Autodesk Inventor part; units mm, degrees
ref_plane "工作平面2" through (-13.4156, -13.4156, 7) normal (0, 0, 1) x (1, -0.0000484, 0)
ref_plane "工作平面3" through (0, 0, 7) normal (0, 0, 1) x (1, 0, 0)
ref_plane "工作平面4" through (-7.4754, -7.4754, 19) normal (0, 0, 1) x (1, -0.0000484, 0)
sketch "草圖1" plane through (0, 0, 0) normal (0, 0, 1) x (1, 0, 0)
  circle A0 centre (0, 0) radius 19.6
  circle A1 centre (0, 0) radius 41.575
  dimension "d0" = 39.2
  dimension "d1" = 83.15
extrude "擠出1" add sketch "草圖1" along normal blind 5
sketch "草圖2" plane through (0, 0, 0) normal (0, 0, -1) x (-1, 0, 0)
  circle A0 centre (0, 0) radius 41.575
extrude "擠出2" add sketch "草圖2" along normal blind 4
sketch "草圖4" plane through (0, 0, 5) normal (0, 0, 1) x (1, 0, 0)
  circle A0 centre (0, 0) radius 41.575
  circle A1 centre (0, 0) radius 37.575
  dimension "d14" = 4
extrude "擠出4" add sketch "草圖4" along normal blind 47.5
sketch "草圖5" plane through (0, 0, 5) normal (0, 0, 1) x (1, 0, 0)
  circle A0 centre (0, 0) radius 37.575
  circle A1 centre (0, 0) radius 33.075
  dimension "d17" = 4.5
extrude "擠出5" add sketch "草圖5" along normal blind 31.5
sketch "草圖6" plane through (0, 0, -4) normal (0, 0, -1) x (-1, 0, 0)
  line L0 (-66.575, 15.075) -> (-66.575, -15.075)
  line L1 (-66.575, 15.075) -> (-38.7456, 15.075)
  circle A0 centre (0, 0) radius 41.575
  line L2 (-66.575, -15.075) -> (-38.7456, -15.075)
  point P0 (-41.575, 0)
  dimension "d20" = 30.15
  dimension "d22" = 15.075
  dimension "d25" = 25
extrude "擠出6" add sketch "草圖6" against normal up to surface (56.5 mm away) contours L1 A0 L2 L0
sketch "草圖7" plane through (66.575, -15.075, -4) normal (1, 0, 0) x (0, 0, -1)
  line L0 (-56.5, 30.15) -> (-56.5, 0)
  line L1 (0, 0) -> (-56.5, 0)
  line L2 (0, 30.15) -> (0, 0)
  line L3 (0, 30.15) -> (-56.5, 30.15)
  line L4 (-51.5, 5) -> (-31.35, 5)
  line L5 (-31.35, 5) -> (-31.35, 25.15)
  line L6 (-31.35, 25.15) -> (-51.5, 25.15)
  line L7 (-51.5, 25.15) -> (-51.5, 5)
  line L8 (-51.5, 5) -> (-31.35, 25.15) construction
  line L9 (-31.35, 5) -> (-51.5, 25.15) construction
  line L10 (-25.15, 5.0185) -> (-5, 5.0185)
  line L11 (-5, 5.0185) -> (-5, 25.15)
  line L12 (-5, 25.15) -> (-25.15, 25.15)
  line L13 (-25.15, 25.15) -> (-25.15, 5.0185)
  line L14 (-25.15, 5.0185) -> (-5, 25.15) construction
  line L15 (-5, 5.0185) -> (-25.15, 25.15) construction
  point P0 (-4, 15.075)
  point P1 (-41.425, 15.075)
  point P2 (-15.075, 15.0842)
  dimension "d26" = 20.15
  dimension "d27" = 20.15
  dimension "d28" = 20.15
  dimension "d29" = 5
  dimension "d30" = 5
  dimension "d31" = 5
extrude "擠出7" cut sketch "草圖7" against normal blind 20 contours L7 L6 L5 L4 | L13 L12 L11 L10
fillet "圓角1" radius 2 7 edges at (52.6603, 15.075, -4) (-41.575, 0, -4) (52.6603, -15.075, -4) (38.7456, 15.075, 24.25) (52.6603, 15.075, 52.5) (-41.575, 0, 52.5) (52.6603, -15.075, 52.5)
sketch "草圖8" plane through (0, 0, 52.5) normal (0, 0, 1) x (1, 0, 0)
  line L0 (52.9465, -6.0747) -> (44.9865, -6.0635)
  line L1 (52.9465, -6.0747) -> (52.9551, 0.0253)
  line L2 (44.9951, 0.0365) -> (52.9551, 0.0253)
  line L3 (44.9865, -6.0635) -> (44.9951, 0.0365)
  circle A0 centre (48.975, -7.075) radius 2.165
  circle A1 centre (48.975, 7.075) radius 2.165
  line L4 (38.7456, -15.075) -> (66.575, -15.075)
  line L5 (66.575, 15.075) -> (40.0902, 15.075)
  point P0 (0, 0)
  dimension "d36" = 4.33
  dimension "d37" = 4.33
  dimension "d38" = 8
  dimension "d39" = 8
extrude "擠出8" cut sketch "草圖8" against normal up to surface (5 mm away) contours A0 L0 | L0 A0 | A1
sketch "草圖9" plane through (38.7456, -15.075, 50.5) normal (0, -1, 0) x (1, 0, 0)
  line L0 (27.8294, -29.35) -> (27.8294, -49.5)
  line L1 (27.8294, -29.35) -> (7.8294, -29.35)
  line L2 (7.8294, -29.35) -> (7.8294, -49.5)
  line L3 (27.8294, -49.5) -> (7.8294, -49.5)
  line L4 (27.8294, -3) -> (27.8294, -23.15)
  line L5 (27.8294, -3) -> (7.8294, -3)
  line L6 (7.8294, -3) -> (7.8294, -23.15)
  line L7 (27.8294, -23.15) -> (7.8294, -23.15)
  circle A0 centre (17.8294, -39.425) radius 2.1
  circle A1 centre (17.8294, -13.075) radius 2.1
  point P0 (-38.7456, -50.5)
  dimension "d42" = 4.2
  dimension "d43" = 4.2
extrude "擠出9" cut sketch "草圖9" against normal through all contours A0 | A1
sketch "草圖10" plane through (38.7456, -15.075, 50.5) normal (0, -1, 0) x (1, 0, 0)
  circle A0 centre (17.8294, -39.425) radius 2.1
  circle A1 centre (17.8294, -39.425) radius 3.65
  circle A2 centre (17.8294, -13.075) radius 2.1
  circle A3 centre (17.8294, -13.075) radius 3.65
  point P0 (-38.7456, -50.5)
  dimension "d46" = 7.3
  dimension "d47" = 7.3
extrude "擠出10" cut sketch "草圖10" against normal blind 3
mirror "鏡射1" about plane through (0, 0, 0) normal (0, 1, 0) of "擠出10"
sketch "草圖14" plane through (0, 0, 5) normal (0, 0, 1) x (1, 0, 0)
  circle A0 centre (0, 0) radius 19.6
extrude "擠出13" add sketch "草圖14" against normal up to surface (9 mm away)
sketch "草圖15" plane through (0, 0, -4) normal (0, 0, -1) x (-1, 0, 0)
  circle A0 centre (0, 0) radius 13.5
  dimension "d64" = 27
extrude "擠出14" cut sketch "草圖15" against normal up to surface (9 mm away)
sketch "草圖16" plane through (0, 0, 5) normal (0, 0, 1) x (1, 0, 0)
  circle A0 centre (0, 0) radius 18.415
  circle A1 centre (0, 0) radius 13.5
ref_plane "工作平面2" through (-13.4156, -13.4156, 7) normal (0, 0, 1) x (1, -0.0000484, 0)
extrude "擠出15" add sketch "草圖16" along normal up to surface (2 mm away)
ref_plane "工作平面3" through (0, 0, 7) normal (0, 0, 1) x (1, 0, 0)
sketch "草圖17" plane through (0, 0, 7) normal (0, 0, 1) x (1, 0, 0)
  circle A0 centre (0, 0) radius 7.575
  circle A1 centre (0, 0) radius 18.415
  dimension "d71" = 15.15
extrude "擠出16" add sketch "草圖17" along normal blind 3
sketch "草圖18" plane through (0, 0, 10) normal (0, 0, 1) x (1, 0, 0)
  circle A0 centre (0, 0) radius 7.575
  circle A1 centre (0, 0) radius 10.575
  point P0 (0, 0)
  dimension "d74" = 3
ref_plane "工作平面4" through (-7.4754, -7.4754, 19) normal (0, 0, 1) x (1, -0.0000484, 0)
extrude "擠出17" add sketch "草圖18" along normal up to surface (9 mm away)
fillet "圓角3" radius 3 2 edges at (-18.415, 0, 5) (-10.575, 0, 10)
chamfer "倒角1" distance 1 angle 45 1 edges at (13.5, 0, -4)
equation "\"d27\" = d26"
equation "\"d28\" = d26"
properties part number "j2 arm part_3D 列印"
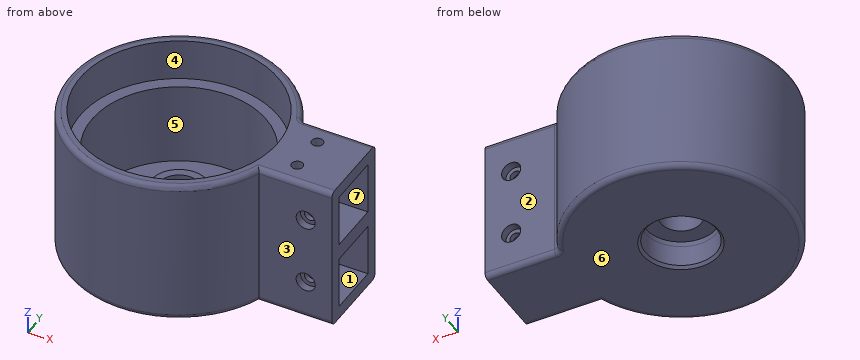
Source: CAD feature listing. Evaluate the final solid. Frame: model axes, mm. Face numbers are marked on the shaded views. A direction names the side the tool comes from. Coordinates: 2 decimals unless noted, no trailing zeros. Write each loop counter-clockwise with the first axis right and the second up, starting at its lowest first coordinate (ties: lowest second). Pieces come first, ordered by that corner, then holes. Notation, with made-up numbers: (71, -3) -> (128, -3) arc R25 cw to (128, 30) -> close; hole circle Ø3 at (83, 53.25). An arc over 180 degrees is marked (long way). Return JSON: item names as keys, results as strings. Group by question number.
1) Mould query, pull axis Z, two halves, no side actions, for the marked faces 5, 6 and 7. Classes: +Z half, -Z half, draft (parallel to the pull), parting line (faces both ways), or undercut.
2) Set-up query: the marked faces 1, 2, 3 and 4. Return all of +Z, -Z, +X, -X, +Y, -Y with unobstructed straight access to the full face (end or side cutting, diameter ignored); none if empty.
3) Section query A-A, the plane x = 48.5. State how many separate pieces and enclosed holes the cut face has, plus the area to 3 significant figures.
4) Contact query for flat-ended pins moving along their axis: P1, Ø6, axis at x = 57, z = 11.5, coming from the +Y side (3 decimals); P2, Ø6, axis at x = 57.5, z = 36.5, coming from the +Y side (3 decimals); P3, Ø12, axis at y = -25.5, z = 3, coming from the -X side; P4, Ø3.5, axis at x = 56.575, z = 11.075, coming from the +Y side. Output: stop coordinate, or through.
5) Section query B-B, the plane z = 24. Return loops of the section in (x, y) (3 decimals), plus the area to 3 significant figures.
6) Ray query, line 1 along X through (y, z) = (0, -0.25) (3 decimals); line 2 along Z through (x, y) = (60.5, -2.5); line 3 along Y through (x, z) = (0, 6) (3 decimals). Return the intervals inside material, ascending.
From the geometry:
{
 "1": {"face 5": "draft", "face 6": "-Z half", "face 7": "undercut"},
 "2": {"face 1": "+X", "face 2": "+Z, -Z, +X, +Y", "face 3": "+Z, -Z, +X, -Y", "face 4": "+Z"},
 "3": {"separate pieces": "2", "enclosed holes": "1", "area": "846 mm²"},
 "4": {"P1": "y = 12.075", "P2": "y = 15.075", "P3": "x = -36.72", "P4": "through"},
 "5": {"outline": "(38.25, 16.291) arc R41.575 ccw (long way) to (38.746, -15.075) -> (66.575, -15.075) -> (66.575, 15.075) -> (40.09, 15.075) arc R2 cw to start; hole circle Ø66.15 at (0, 0)", "area": "2,780 mm²"},
 "6": {"line 1": "-41.575 to -13.5, 13.5 to 66.575", "line 2": "-4 to 1, 21.15 to 27.35, 47.5 to 52.5", "line 3": "-41.575 to -33.075, -19.179 to -13.5, 13.5 to 19.179, 33.075 to 41.575"}
}
